Part model, mm, in its own coordinate system. A direction names the side the tool comes from. Give positions to 0.01 mm unless a question says otherwise; leave off trailing zeros. Order: outer loops, then holes, each group sorted by start corner. A loop starts at its lowest first (then second) coordinate and runs counter-clockwise, first axis right, second up.
1. Slice it at C-C on z = 13. List the corners of the cut face in (x, y).
2. Slice it at A-A on y = -20.5. List the corners of the cut face in (x, z), and give its area (3 significant figures).
3. Probe line 1 (Y direction, x = -25, z = 12); line 2 (X direction, y = -33.25, z = 10). List the from-to ranges inside material, lowest first.
4. Which spindle directions (+Z, -Z, +X, -X, +Y, -Y) get a long thin tool onto all of the face, cutting with end or side? Do faces 1 (the flat face through (-20, -33, 14)), 2 (the flat face through (-24.832, -28, 14)). Say none if no direction does.
5. Mould opens along Y. For faces 3 (the flat face through (-29, -33, 9)), 4 (the flat face through (-27, -35.769, 14)), 5 (the flat face through (-28, -17.769, 14)) say: +Y half, -Y half, draft (parallel to the pull), parting line (faces both ways), or undercut.
6. Drop a flat-ended pin along its axis: pin 1 Ø2 at (x, y) = (-25, -25.5) entering from +Z. Give the stop position or say it passes through.
7. Slice it at B-B on x = -25.75. List the corners of the cut face in (y, z).
from build123d import *

# Parameters (mm, degrees)
SKETCH020_W     = 15
SKETCH020_H     = 30
PAD012_DEPTH    = 10
SKETCH023_W     = 3.980878
SKETCH023_H     = 15.550635
POCKET006_DEPTH = 10.001


with BuildPart() as pocket006:
    # Sketch020 → Pad012 (new body)
    with BuildSketch(Plane.XY.offset(9)):
        with Locations((-27.5, 32.769276)):
            Rectangle(SKETCH020_W, SKETCH020_H)
    extrude(amount=PAD012_DEPTH)

    # Sketch023 → Pocket006 (cut, through all)
    with BuildSketch(Plane.XY.offset(19)):
        with Locations((-26.822156, 27.993958)):
            Rectangle(SKETCH023_W, SKETCH023_H)
    extrude(amount=-POCKET006_DEPTH, mode=Mode.SUBTRACT)


with BuildPart() as part_mirroring:
    # Part__Mirroring: instance of Pocket006
    add(pocket006.part.mirror(Plane(origin=(0, 0, 0), x_dir=(1, 0, 0), z_dir=(0, 1, 0))))


solid = part_mirroring.part
Data:
1. outline: (-35, -47.77) - (-20, -47.77) - (-20, -17.77) - (-35, -17.77) - close; hole (-28.81, -35.77) - (-24.83, -35.77) - (-24.83, -20.22) - (-28.81, -20.22) - close
2. outline: (-35, 9) - (-28.81, 9) - (-28.81, 19) - (-35, 19) - close; (-24.83, 9) - (-20, 9) - (-20, 19) - (-24.83, 19) - close
2. area: 110 mm2
3. line 1: y = -47.77 to -35.77, -20.22 to -17.77
3. line 2: x = -35 to -28.81, -24.83 to -20
4. face 1: +Z, -Z, +X, +Y, -Y
4. face 2: +Z, -Z
5. face 3: draft
5. face 4: undercut
5. face 5: +Y half
6. pin 1: stops at z = 19
7. outline: (-47.77, 9) - (-35.77, 9) - (-35.77, 19) - (-47.77, 19) - close; (-20.22, 9) - (-17.77, 9) - (-17.77, 19) - (-20.22, 19) - close
